Could you check a few things on this drawing? It's one solid part, dimensions in mm from its lowest x, y, z. Give positions to 0.01 mm unless a question says otherwise; leave off trailing zeros. Loops run counter-clockwise (first coordinate to the right, second up) from the corner with the lowest first, then second, coordinate; pieces in that order, holes last. Notation, with made-up numbers: (59.25, 52) - (98.25, 52) arc R30 ccw to (98.25, 87) - close; hole circle Ø6 at (-38.75, 25.25). An arc over 180 degrees is marked (long way). Answer as a JSON object with one key per item and string values.
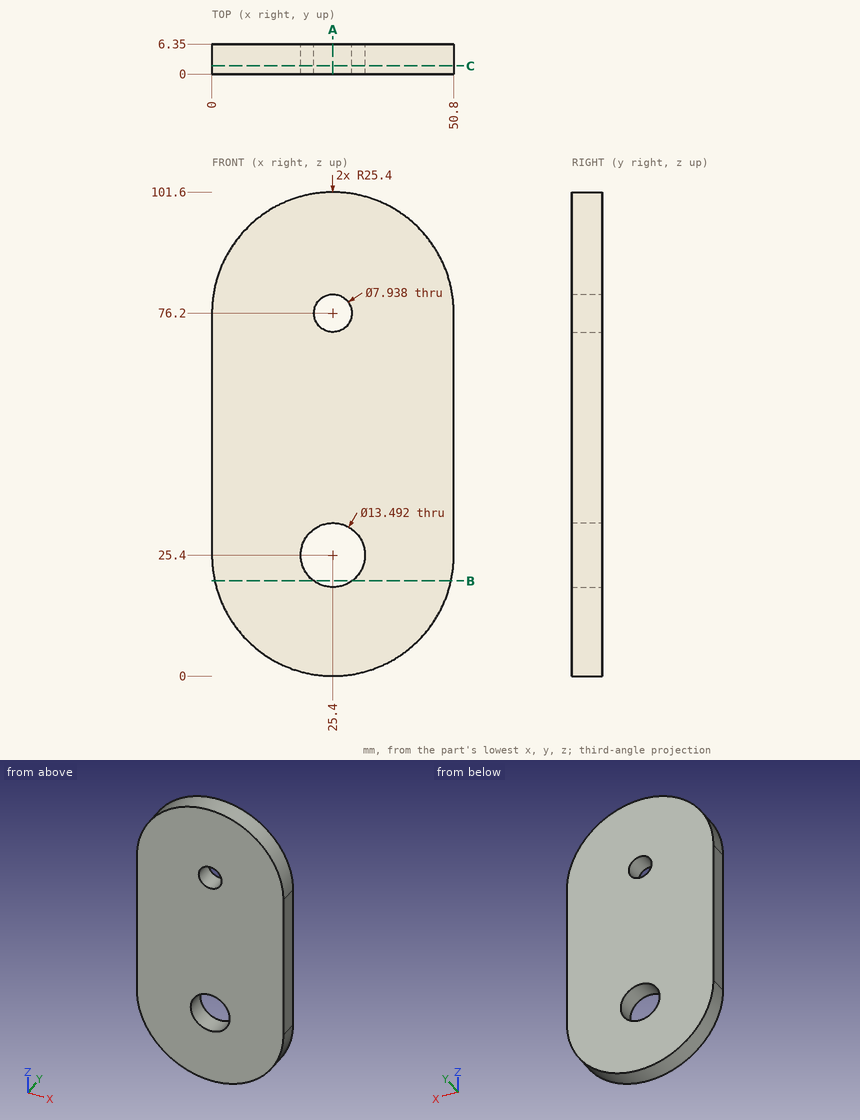
1) Imagine slicing it at C-C on y = 1.75. Write out the boundary of the cut face in (x, z), and give its area (4 significant figures).
Check sheet entries:
{"outline": "(0, 25.4) arc R25.4 ccw to (50.8, 25.4) - (50.8, 76.2) arc R25.4 ccw to (0, 76.2) - close; hole circle Ø13.49 at (25.4, 25.4); hole circle Ø7.94 at (25.4, 76.2)", "area": "4,415 mm2"}
2) Imagine slicing it at B-B on z = 20. Write out the boundary of the cut face in (x, y), and give its area (3 significant figures).
Check sheet entries:
{"outline": "(0.58, 0) - (21.36, 0) - (21.36, 6.35) - (0.58, 6.35) - close; (29.44, 0) - (50.22, 0) - (50.22, 6.35) - (29.44, 6.35) - close", "area": "264 mm2"}
3) Imagine slicing it at A-A on x = 25.4. Write out the boundary of the cut face in (y, z).
Check sheet entries:
{"outline": "(0, 0) - (6.35, 0) - (6.35, 18.65) - (0, 18.65) - close; (0, 32.15) - (6.35, 32.15) - (6.35, 72.23) - (0, 72.23) - close; (0, 80.17) - (6.35, 80.17) - (6.35, 101.6) - (0, 101.6) - close"}
4) I need wall thicknesses on L1, parallel to Z at x = 25.4, y = 3.75; L2, parallel to X at y = 4.25, z = 76.2; L3, parallel to X at y = 3.75, z = 11 (1 decimal). Which ranges of each line are inside material? Lowest first, please.
Check sheet entries:
{"L1": "0 to 18.65, 32.15 to 72.23, 80.17 to 101.6", "L2": "0 to 21.43, 29.37 to 50.8", "L3": "4.5 to 46.3"}
5) I'm going to push flat-ended pins straight in: P1, Ø2, axis at x = 9, y = 4.5, coming from the +Z side; P2, Ø5, axis at x = 25.4, z = 76.2, coming from the -Y side (3 decimals); P3, Ø3, axis at x = 24, y = 4, coming from the +Z side. Where does each tip first touch, or does it pass through?
Check sheet entries:
{"P1": "z = 96.4", "P2": "through", "P3": "z = 101.6"}
